Autodesk Inventor part; units mm, degrees
ref_plane "YZ Plane" through (0, 0, 0) normal (1, 0, 0) x (0, 1, 0)
ref_plane "XZ Plane" through (0, 0, 0) normal (0, 1, 0) x (-1, 0, 0)
ref_plane "XY Plane" through (0, 0, 0) normal (0, 0, 1) x (1, 0, 0)
sketch "Sketch1" plane through (0, 0, 0) normal (0, 1, 0) x (-1, 0, 0)
  circle A0 centre (0, 12.5) radius 2.6
  circle A1 centre (0, -12.5) radius 2.6
  circle A2 centre (0, 12.5) radius 4.75
  circle A3 centre (0, -12.5) radius 4.75
  circle A4 centre (0, 12.5) radius 7.5
  circle A5 centre (0, -12.5) radius 7.5
  line L0 (7.5, 12.5) -> (7.5, -12.5)
  line L1 (-7.5, -12.5) -> (-7.5, 12.5)
  line L2 (0, 12.5) -> (0, -12.5) construction
  line L3 (7.5, -12.5) -> (7.5, 12.5)
  line L4 (-10, 41) -> (10, 41)
  line L5 (10, 41) -> (10, -41)
  line L6 (10, -41) -> (-10, -41)
  line L7 (-10, -41) -> (-10, 41)
  point P0 (0, 0)
  dimension "d0" = 5.2
  dimension "d1" = 5.2
  dimension "d2" = 25
  dimension "d3" = 12.5
  dimension "d6" = 9.5
  dimension "d7" = 9.5
  dimension "d8" = 15
  dimension "d9" = 15
  dimension "d19" = 20
  dimension "d20" = 82
  dimension "d21" = 41
  dimension "d38" = 10
extrude "Extrusion1" add sketch "Sketch1" along normal blind 3 contours A2 | A3
extrude "Extrusion2" add sketch "Sketch1" along normal blind 7 contours A4 | L0 A5 L1 A4 | A5 | L4 L5 L6 L7
sketch "Sketch2" plane through (0, 7, 0) normal (0, 1, 0) x (1, 0, 0)
  circle A0 centre (0, 12.5) radius 4.75
  circle A1 centre (0, -12.5) radius 4.75
  line L0 (-10, -41) -> (10, -41)
  line L1 (10, -41) -> (10, 41)
  line L2 (10, 41) -> (-10, 41)
  line L3 (-10, 41) -> (-10, -41)
  line L4 (10, 41) -> (10, -41)
  line L5 (10, -37) -> (-10, -37)
  line L6 (10, 37) -> (-10, 37)
  point P0 (0, 0)
  dimension "d24" = 4
  dimension "d25" = 4
extrude "Extrusion3" add sketch "Sketch2" along normal blind 8.4 contours L3 L5 L1 L0 | L3 L2 L1 L6
sketch "Sketch3" plane through (0, 15.4, 0) normal (0, 1, 0) x (1, 0, 0)
  line L0 (10, 41) -> (-10, 41)
  line L1 (-10, 41) -> (-10, 37)
  line L2 (-10, -41) -> (10, -41)
  line L3 (10, 37) -> (10, 41)
  line L4 (-10, 37) -> (10, 37)
  line L5 (10, -41) -> (10, -37)
  line L6 (10, -37) -> (-10, -37)
  line L7 (-10, -37) -> (-10, -41)
  line L8 (-10, -41) -> (10, -41)
  line L9 (10, -41) -> (10, -32.8)
  line L10 (10, -32.8) -> (-10, -32.8)
  line L11 (-10, -32.8) -> (-10, -41)
  line L12 (10, -37) -> (10, 37)
  line L13 (-10, 41) -> (10, 41)
  line L14 (10, 41) -> (10, 32.8)
  line L15 (10, 32.8) -> (-10, 32.8)
  line L16 (-10, 32.8) -> (-10, 41)
  dimension "d39" = 4.2
  dimension "d40" = 4.2
extrude "Extrusion4" add sketch "Sketch3" along normal blind 3
fillet "Fillet4" radius 4 2 edges at (0, 7, 37) (0, 7, -37)
fillet "Fillet5" radius 4.2 2 edges at (0, 15.4, -37) (0, 15.4, 37)
fillet "Fillet6" radius 2 2 edges at (0, 18.4, 32.8) (0, 18.4, -32.8)
fillet "Fillet7" radius 10 2 edges at (0, 0, 41) (0, 0, -41)
fillet "Fillet8" radius 8.25 2 edges at (0, 18.4, 41) (0, 18.4, -41)
fillet "Fillet9" radius 2 14 edges at (10, 8.1716, -35.8284) (10, 11.1, -37) (10, 14.1699, -35.7699) (10, 8.1716, 35.8284) (10, 11.1, 37) (10, 14.1699, 35.7699) (10, 7, 0) (-10, 8.1716, 35.8284) (-10, 11.1, 37) (-10, 14.1699, 35.7699) (-10, 8.1716, -35.8284) (-10, 11.1, -37) (-10, 14.1699, -35.7699) (-10, 7, 0)
properties part number "HolderMid"
Read the model definition and answer for the solid it produces. Units are mm, in the model's axes. A direction names the side the tool comes from. Round coordinates to 2 decimals unless told otherwise and drop trailing zeros. Write each loop counter-clockwise with the first axis right and the second up, starting at its lowest first coordinate (ties: lowest second). Pieces come first, ordered by that corner, then holes. Notation, with made-up numbers: (30.25, 21.5) - (88.25, 21.5) arc R18 ccw to (88.25, 32.5) - close; hole circle Ø11 at (-10, -24.75). An arc over 180 degrees is marked (long way). Use CSV: the item, a comma, the result in double quotes.
Q1. Find section D-D, the plane x = 0. Count the separate pieces of the cut face and the enclosed holes in it, then the cut area to 3 significant figures.
Values:
separate pieces,"3"
enclosed holes,"0"
area,"527 mm²"
Q2. A tool of negligible diameter and unlimited length cuts with its end or side. For faces 5 (the flat face through (10, 4, 0)), 6 (the cylindrical face through (0.14, 2.85, -37.99)), 7 (the cylindrical face through (-0.11, 14.14, 35.8)), 8 (the flat face through (-2, 3, 10)), 9 (the cylindrical face through (-0.14, 17.83, 33.4)), from which of +Z, -Z, +X, -X, +Y, -Y can it reach the whole face along a straight path? Write none if from no direction.
Values:
face 5,"+Z, -Z, +X, +Y, -Y"
face 6,"-Z, +X, -X, -Y"
face 7,"+X, -X"
face 8,"+Y"
face 9,"+X, -X, +Y"
Q3. Find section A-A, the plane z = -12.5. Write down the section's boundary in (x, y), then the cut area to 3 significant figures.
Values:
outline,"(-10, 0) - (-2.6, 0) - (-2.6, 3) - (-4.75, 3) - (-4.75, 7) - (-8, 7) arc R2 ccw to (-10, 5) - close; (2.6, 0) - (10, 0) - (10, 5) arc R2 ccw to (8, 7) - (4.75, 7) - (4.75, 3) - (2.6, 3) - close"
area,"84.7 mm²"
Q4. Each of these flat-tipped pins is pushed along its axis until it touches: pin 1 Ø10.5 at (x, z) = (2.5, 11) entering from +Y; pin 2 Ø0.8 at (x, y) = (-3.5, 16) entering from +Z; pin 3 Ø7.5 at (x, z) = (0.5, -12.5) entering from +Y. Where does it stop, or does it pass through?
Values:
pin 1,"stops at y = 7"
pin 2,"stops at z = 39.16"
pin 3,"stops at y = 3"
Q5. Find section C-C, the plane z = 25. Write down the section's boundary in (x, y), then the cut area to 3 significant figures.
Values:
outline,"(-10, 0) - (10, 0) - (10, 5) arc R2 ccw to (8, 7) - (-8, 7) arc R2 ccw to (-10, 5) - close"
area,"138 mm²"
Q6. Determine the mould class of faces 1 (the cylindrical face through (-0.112, 8.141, 35.797)), 2 (the cylindrical face through (-4.53, 4.97, 11.07)), 3 (the flat face through (0, 0, 0)), 4 (the cylindrical face through (-0.14, 15.41, 39.31)) for opening direction Y: +Y half, -Y half, draft (parallel to the pull), parting line (faces both ways), or undercut.
Values:
face 1,"undercut"
face 2,"draft"
face 3,"-Y half"
face 4,"+Y half"
Q7. Straight lines are drawn through the part: line 1 along Z through (x, y) = (0, 1.6); line 2 along Z through (x, y) = (0, 2); line 3 along Y through (x, z) = (-5.5, -20). For each, find the intervals that lie inside material, in ascending order.
Values:
line 1,"z = -36.43 to -15.1, -9.9 to 9.9, 15.1 to 36.43"
line 2,"z = -37 to -15.1, -9.9 to 9.9, 15.1 to 37"
line 3,"y = 0 to 7"
